Input: part model. Units: mm. Frame: model coordinates. Face numbers are marked on the shaded views. A direction names the side the tool comes from. Round coordinates to 2 decimals unless told otherwise and drop trailing zeros. Loops run counter-clockwise (first coordinate to the right, second up) from the corner with the lowest first, then second, coordinate; pieces in that order, holes last. Notation, with made-up numbers: M -5,-34 L 45,-34 A14 ccw 45,-28 Z; hole C 85,78.25 d11. An arc over 180 degrees is marked long. Put each result on its own line as item: value. Start each with the question number.
1) Pin query (flat end, axial travel): pin 1 (1 mm diameter, centred on x = -7, y = -1.5, fed in from +Z); pin 2 (0.8 mm diameter, centred on x = 5, y = 0.5, fed in from -Z); pin 3 (1.8 mm diameter, centred on x = -16.75, z = 0, fed in from +Y); pin 4 (2.5 mm diameter, centred on x = 7.75, z = 0, fed in from -Y). Return the tip coordinate at first contact, or that it passes through.
2) Section C-C on y = 2.25. Output: boundary loops of the cut face in (x, z).
3) Section A-A on x = 7.75. Output: boundary loops of the cut face in (y, z), plus the area to 3 significant figures.
4) Reachability of the marked faces 5, 6, 7, 8 and 9 from +Z, -Z, +X, -X, +Y, -Y: full face, straight path, thin tool, end or side. Return the list, or none.
5) Line query: probe 1 along X at (y, z) = (3.4, 0); probe 2 along Y at (x, z) = (6.5, -2); probe 3 along X at (y, z) = (3, 1.25). Output: solid intervals per line, ascending.
6) Draft query along X for the marked faces 1, 2, 3 and 4. Return one class per face: +X half, -X half, draft (parallel to the pull), parting line (faces both ways), or undercut.
7) Section B-B on y = -0.5. State how many separate pieces and enclosed holes the cut face has, plus the area to 3 significant figures.
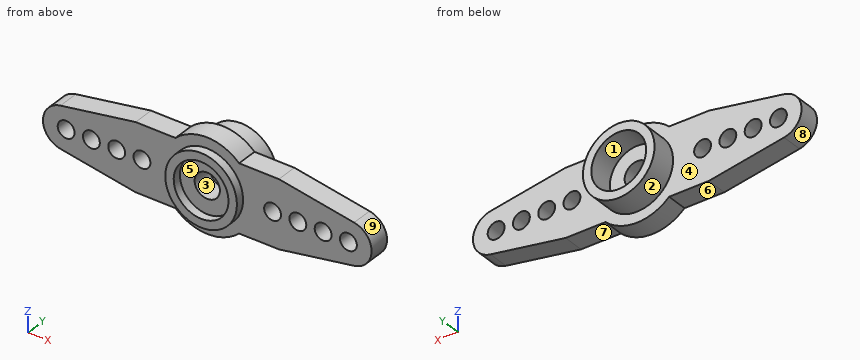
from build123d import *

# Parameters (mm, degrees)
SKETCH1_R                = 1
SKETCH1_R_2              = 1.5
BOSS_EXTRUDE1_DEPTH      = 1.25
BOSS_EXTRUDE2_DEPTH      = 3
BOSS_EXTRUDE2_DEPTH_BACK = 3.5
BOSS_EXTRUDE2_START      = 1.25
SKETCH3_R                = 4.25
SKETCH3_R_2              = 3.25


with BuildPart() as part:
    # Sketch1 → Boss-Extrude1 (new, symmetric)
    # profile 1 of 3: a face of its own
    with BuildSketch(Plane(origin=(0, 0, 0), x_dir=(1, 0, 0), z_dir=(0, 1, 0))):
        with BuildLine():
            ThreePointArc((17.424122962, 2.463761294), (19.5, 0), (17.424122962, -2.463761294))
            Line((17.424122962, -2.463761294), (8.5, -4))
            Line((8.5, -4), (-8.5, -4))
            Line((-8.5, -4), (-17.424122962, -2.463761294))
            ThreePointArc((-17.424122962, -2.463761294), (-19.5, 0), (-17.424122962, 2.463761294))
            Line((-17.424122962, 2.463761294), (-8.5, 4))
            Line((-8.5, 4), (8.5, 4))
            Line((8.5, 4), (17.424122962, 2.463761294))
        make_face()
        with Locations(Location((-7.75, 0, 0), (0, 0, 270))):
            Circle(SKETCH1_R, mode=Mode.SUBTRACT)
        with Locations(Location((-16.75, 0, 0), (0, 0, 270))):
            Circle(SKETCH1_R, mode=Mode.SUBTRACT)
        with Locations(Location((16.75, 0, 0), (0, 0, 270))):
            Circle(SKETCH1_R, mode=Mode.SUBTRACT)
        with Locations(Location((13.75, 0, 0), (0, 0, 270))):
            Circle(SKETCH1_R, mode=Mode.SUBTRACT)
        with Locations(Location((10.75, 0, 0), (0, 0, 270))):
            Circle(SKETCH1_R, mode=Mode.SUBTRACT)
        with Locations(Location((7.75, 0, 0), (0, 0, 270))):
            Circle(SKETCH1_R, mode=Mode.SUBTRACT)
        with Locations(Location((0, 0, 0), (0, 0, 270))):
            Circle(SKETCH1_R_2, mode=Mode.SUBTRACT)
        with Locations(Location((-13.75, 0, 0), (0, 0, 270))):
            Circle(SKETCH1_R, mode=Mode.SUBTRACT)
        with Locations(Location((-10.75, 0, 0), (0, 0, 270))):
            Circle(SKETCH1_R, mode=Mode.SUBTRACT)
    # profile 2 of 3: a face of its own
    with BuildSketch(Plane(origin=(0, 0, 0), x_dir=(1, 0, 0), z_dir=(0, 1, 0))):
        with BuildLine():
            ThreePointArc((3.774917218, 4), (0, 5.5), (-3.774917218, 4))
            Line((-3.774917218, 4), (3.774917218, 4))
        make_face()
    # profile 3 of 3: a face of its own
    with BuildSketch(Plane(origin=(0, 0, 0), x_dir=(1, 0, 0), z_dir=(0, 1, 0))):
        with BuildLine():
            Line((3.774917218, -4), (-3.774917218, -4))
            ThreePointArc((-3.774917218, -4), (0, -5.5), (3.774917218, -4))
        make_face()
    extrude(amount=BOSS_EXTRUDE1_DEPTH, both=True)

    # Sketch3 → Boss-Extrude2 (add, two sides: drawn at the far end of the back side and taken through both)
    with BuildSketch(Plane(origin=(0, 0, 0), x_dir=(1, 0, 0), z_dir=(0, 1, 0)).offset(BOSS_EXTRUDE2_START - BOSS_EXTRUDE2_DEPTH_BACK)):
        with Locations(Location((0, 0, 0), (0, 0, 270))):
            Circle(SKETCH3_R)
        with Locations(Location((0, 0, 0), (0, 0, 270))):
            Circle(SKETCH3_R_2, mode=Mode.SUBTRACT)
    extrude(amount=BOSS_EXTRUDE2_DEPTH + BOSS_EXTRUDE2_DEPTH_BACK)


solid = part.part
Geometry results:
1. pin 1: stops at z = 4
1. pin 2: stops at z = -4
1. pin 3: passes through
1. pin 4: stops at y = -1.25
2. outline: C 0,0 d8.5; hole C 0,0 d6.5
3. outline: M -1.25,-4 L 1.25,-4 L 1.25,-1 L -1.25,-1 Z; M -1.25,1 L 1.25,1 L 1.25,4 L -1.25,4 Z
3. area: 15.0 mm²
4. face 5: -Y
4. face 6: -Z, -X, +Y, -Y
4. face 7: -Z, +X, +Y, -Y
4. face 8: -X, +Y, -Y
4. face 9: +X, +Y, -Y
5. probe 1: x = -4.25 to -3.25, 3.25 to 4.25
5. probe 2: y = -1.25 to 1.25
5. probe 3: x = -4.06 to -3, 3 to 4.06
6. face 1: undercut
6. face 2: parting line
6. face 3: undercut
6. face 4: draft
7. separate pieces: 1
7. enclosed holes: 9
7. area: 250 mm²
